```python
from build123d import *

# Parameters (mm, degrees)
BOSS_EXTRUDE1_DEPTH = 6
BOSS_EXTRUDE2_DEPTH = 3
BOSS_EXTRUDE3_DEPTH = 6


with BuildPart() as part:
    # Sketch1 → Boss-Extrude1 (new body)
    with BuildSketch(Plane.XY):
        Polygon((0, 8.1), (-7.014805771, 4.05), (-7.014805771, -4.05), (0, -8.1), (7.014805771, -4.05), (7.014805771, 4.05), align=None)
    extrude(amount=BOSS_EXTRUDE1_DEPTH)

    # Sketch2 → Boss-Extrude2 (add)
    with BuildSketch(Plane(origin=(0, 0, 0), x_dir=(-1, 0, 0), z_dir=(0, 0, -1))):
        Polygon((0, 8.1), (0, -8.1), (-7.014805771, -4.05), (-7.014805771, 4.05), align=None)
        Polygon((0, 8.1), (0, -8.1), (7.014805771, -4.05), (7.014805771, 4.05), align=None)
        Polygon((0, 8.1), (-28.5, 8.1), (-28.5, -8.1), (0, -8.1), (-7.014805771, -4.05), (-7.014805771, 4.05), align=None)
        Polygon((-28.5, 8.1), (-57, 8.1), (-49.985194229, 4.05), (-49.985194229, -4.05), (-57, -8.1), (-28.5, -8.1), align=None)
        Polygon((-57, 8.1), (-49.985194229, 4.05), (-49.985194229, -4.05), (-57, -8.1), align=None)
        Polygon((-57, 8.1), (-57, -8.1), (-64.014805771, -4.05), (-64.014805771, 4.05), align=None)
    extrude(amount=BOSS_EXTRUDE2_DEPTH)

    # Sketch3 → Boss-Extrude3 (add)
    with BuildSketch(Plane.XY):
        Polygon((64.014805771, -4.05), (64.014805771, 4.05), (57, 8.1), (49.985194229, 4.05), (49.985194229, -4.05), (57, -8.1), align=None)
    extrude(amount=BOSS_EXTRUDE3_DEPTH)


solid = part.part
```
For this review, take the finished solid that the model builds, in its own axes (mm). A direction names the side the tool comes from. Coordinates: 2 decimals unless noted, no trailing zeros. Loops run counter-clockwise (first coordinate to the right, second up) from the corner with the lowest first, then second, coordinate; pieces in that order, holes last.
1. Add section C-C, the plane x = 1.5. Give the boundary of the cut face in (y, z).
2. Add section D-D, the plane x = 11.5. Give the boundary of the cut face in (y, z).
3. Mouldability with a two-part tool opening along X and no side actions: class faces 5 (the flat face through (28, 0, 0)), 6 (the flat face through (-7.015, 0, 2)), 7 (the flat face through (57, 0, 6)), 8 (the flat face through (60.458, -6.103, 1.437)) as +X half, -X half, draft (parallel to the pull), parting line (faces both ways), or undercut.
4. For line 1 (X direction, y = 3.75, z = 0.5); line 2 (X direction, y = -5, z = 0.75); line 3 (Z direction, x = 43.5, y = 6.75), list the stretches that pass through material, from the lowest coordinate up.
5. For faces 1 (the flat face through (28, 0, -3)), 2 (the flat face through (53.443, -6.047, 2.958)), 3 (the flat face through (53.542, 6.103, 2.958)), 4 (the flat face through (49.985, 0, 3)), list the 3-axis set-ups (+Z, -Z, +X, -X, +Y, -Y) from which the entire face can be reached by the end or side of a thin tool; tool diameter is ignored.
6. Add section B-B, the plane y = 1. Give the boundary of the cut face in (x, z), then the cut area to 3 significant figures.
7. Insertion check: P1, Ø5, axis at x = 8, y = -2.5, coming from the +Z side; P2, Ø8, axis at x = 26, y = -3.5, coming from the +Z side. Each pin has a flat end and moves straight along its axis. Give the tip position at first contact, or say it passes through.
8. Add section A-A, the plane z = 1.25. Give the boundary of the cut face in (x, y).
Result:
1. outline: (-8.1, -3) - (8.1, -3) - (8.1, 0) - (7.23, 0) - (7.23, 6) - (-7.23, 6) - (-7.23, 0) - (-8.1, 0) - close
2. outline: (-8.1, -3) - (8.1, -3) - (8.1, 0) - (-8.1, 0) - close
3. face 5: undercut
3. face 6: -X half
3. face 7: draft
3. face 8: +X half
4. line 1: x = -7.01 to 7.01, 49.99 to 64.01
4. line 2: x = -5.37 to 5.37, 51.63 to 62.37
4. line 3: z = -3 to 0
5. face 1: -Z, +X, -X, +Y, -Y
5. face 2: +Z, -Y
5. face 3: +Z, +Y
5. face 4: +Z, +Y, -Y
6. outline: (-7.01, -3) - (64.01, -3) - (64.01, 6) - (49.99, 6) - (49.99, 0) - (7.01, 0) - (7.01, 6) - (-7.01, 6) - close
6. area: 381 mm2
7. P1: stops at z = 6
7. P2: stops at z = 0
8. outline: (-7.01, -4.05) - (0, -8.1) - (7.01, -4.05) - (7.01, 4.05) - (0, 8.1) - (-7.01, 4.05) - close; (49.99, -4.05) - (57, -8.1) - (64.01, -4.05) - (64.01, 4.05) - (57, 8.1) - (49.99, 4.05) - close
